Could you check a few things on this model? Use its own coordinates, in mm. A direction names the side the tool comes from. Give positions to 0.01 mm unless a question says otherwise; leave off trailing zeros. Loops run counter-clockwise (first coordinate to the right, second up) from the corner with the lowest first, then second, coordinate; pieces in that order, holes last. Notation, with made-up numbers: M 51,-9.5 L 82,-9.5 A9 ccw 82,7.5 Z; hole C 38.5,-28 d3. An arc over 180 degrees is marked long. Use a Markdown table: item, result. Add a question column.
1) We'd pull the mould along Z, two halves only. Please class faces 5 (the cylindrical face through (4.45, 1.01, 6.43)), 6 (the cylindrical face through (4.45, 39.83, -2.57)), 7 (the flat face through (15, 1, -7)), 8 (the flat face through (8, 22, -4)): +Z half, -Z half, draft (parallel to the pull), parting line (faces both ways), or undercut.
2) If I drill on line 1 along X through (y, z) = (0.9, -4); line 2 along X through (y, z) = (38.85, -4); line 3 along X through (y, z) = (28, -1.5), over which ranges is the centre line in solid material (lowest first)? Write a range as [from, to].
3) Suppose I cut it at B-B on x = 4. List the corners of the cut face in (y, z) for me, and give its area (3 significant figures).
4) Suppose I cut it at A-A on z = -4. List the corners of the cut face in (x, y) for me, and give its area (3 significant figures).
5) Suppose I cut it at C-C on z = 5. List the corners of the cut face in (x, y) for me.
6) Will these pins go through, and if not, where does the flat tip stop? pin 1 Ø9 at (x, y) = (3.5, 19) entering from +Z; pin 2 Ø6.5 at (y, z) = (16, -4) entering from +X; pin 3 Ø1 at (x, z) = (2.5, 3) entering from +Y.
7) Which directions (+Z, -Z, +X, -X, +Y, -Y) give clear straight access to the entire face, cutting with the end or side of a thin tool? Please do faces 1 (the flat face through (11, 2, -4)), 2 (the flat face through (8, 1, 3)), 3 (the flat face through (4, 2, 3)), 4 (the flat face through (4, 37.8, -4)).
8) Suppose I cut it at D-D on x = 13. List the corners of the cut face in (y, z) for me.
```python
from build123d import *

# Parameters (mm, degrees)
SKETCH1_W           = 8
SKETCH1_H           = 8
BOSS_EXTRUDE1_DEPTH = 41.8
SKETCH2_R           = 1.5
CUT_EXTRUDE1_DEPTH  = 4
SKETCH3_W           = 8
SKETCH3_H           = 8
BOSS_EXTRUDE2_DEPTH = 2
SKETCH4_W           = 8
SKETCH4_H           = 8
BOSS_EXTRUDE3_DEPTH = 2
CHAMFER1_SIZE       = 2
SKETCH5_R           = 1.5
CUT_EXTRUDE2_DEPTH  = 2


with BuildPart() as part:
    # Sketch1 → Boss-Extrude1 (new body)
    with BuildSketch(Plane(origin=(0, 0, 0), x_dir=(1, 0, 0), z_dir=(0, 1, 0))):
        with Locations((4, 4)):
            Rectangle(SKETCH1_W, SKETCH1_H)
    extrude(amount=BOSS_EXTRUDE1_DEPTH)

    # Sketch2 → Cut-Extrude1 (cut)
    with BuildSketch(Plane(origin=(0, 41.8, 0), x_dir=(1, 0, 0), z_dir=(0, 1, 0))):
        with Locations(Location((4, 4, 0), (0, 0, 270))):
            Circle(SKETCH2_R)
    extrude(amount=-CUT_EXTRUDE1_DEPTH, mode=Mode.SUBTRACT)

    # Sketch3 → Boss-Extrude2 (add)
    with BuildSketch(Plane(origin=(0, 0, 0), x_dir=(1, 0, 0), z_dir=(0, 1, 0))):
        with Locations((12, 4)):
            Rectangle(SKETCH3_W, SKETCH3_H)
    extrude(amount=BOSS_EXTRUDE2_DEPTH)

    # Sketch4 → Boss-Extrude3 (add)
    with BuildSketch(Plane(origin=(0, 0, 0), x_dir=(1, 0, 0), z_dir=(0, 1, 0))):
        with Locations((4, -4)):
            Rectangle(SKETCH4_W, SKETCH4_H)
    extrude(amount=BOSS_EXTRUDE3_DEPTH)

    # Chamfer1
    chamfer1_edges = [part.edges().sort_by_distance(p)[0] for p in [
        (16, 1, 0),
        (16, 1, -8),
        (0, 1, 8),
        (8, 1, 8),
    ]]
    chamfer(chamfer1_edges, length=CHAMFER1_SIZE)

    # Sketch5 → Cut-Extrude2 (cut)
    with BuildSketch(Plane(origin=(0, 2, 0), x_dir=(1, 0, 0), z_dir=(0, 1, 0))):
        with Locations(Location((4, -5, 0), (0, 0, 270))):
            Circle(SKETCH5_R)
        with Locations(Location((13, 4, 0), (0, 0, 270))):
            Circle(SKETCH5_R)
    extrude(amount=-CUT_EXTRUDE2_DEPTH, mode=Mode.SUBTRACT)


solid = part.part
```
Answer block:
| question | item | result |
|---|---|---|
| 1 | face 5 | undercut |
| 1 | face 6 | undercut |
| 1 | face 7 | -Z half |
| 1 | face 8 | draft |
| 2 | line 1 | x = [0, 11.5], [14.5, 16] |
| 2 | line 2 | x = [0, 2.5], [5.5, 8] |
| 2 | line 3 | x = [0, 8] |
| 3 | outline | M 0,-8 L 41.8,-8 L 41.8,-5.5 L 37.8,-5.5 L 37.8,-2.5 L 41.8,-2.5 L 41.8,0 L 2,0 L 2,3.5 L 0,3.5 Z; M 0,6.5 L 2,6.5 L 2,8 L 0,8 Z |
| 3 | area | 332 mm^2 |
| 4 | outline | M 0,0 L 11.5,0 L 11.5,2 L 8,2 L 8,41.8 L 5.5,41.8 L 5.5,37.8 L 2.5,37.8 L 2.5,41.8 L 0,41.8 Z; M 14.5,0 L 16,0 L 16,2 L 14.5,2 Z |
| 4 | area | 332 mm^2 |
| 5 | outline | M 0,0 L 2.5,0 L 2.5,2 L 0,2 Z; M 5.5,0 L 8,0 L 8,2 L 5.5,2 Z |
| 6 | pin 1 | stops at z = 0 |
| 6 | pin 2 | stops at x = 8 |
| 6 | pin 3 | stops at y = 2 |
| 7 | face 1 | +Z, -Z, +X, +Y |
| 7 | face 2 | +Z, +X, +Y, -Y |
| 7 | face 3 | +Z, +X, -X, +Y |
| 7 | face 4 | +Y |
| 8 | outline | M 0,-8 L 2,-8 L 2,-5.5 L 0,-5.5 Z; M 0,-2.5 L 2,-2.5 L 2,0 L 0,0 Z |
